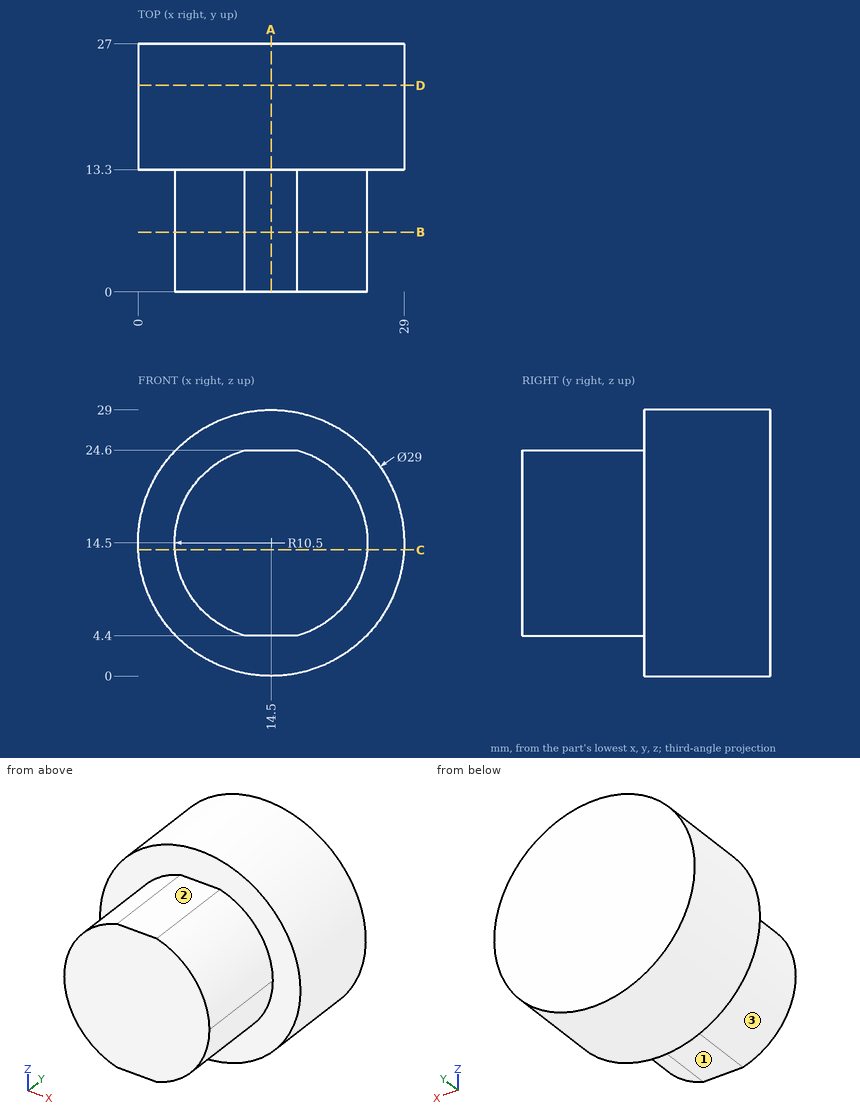
Check sheet for the drawn part. Datum: minimum x, y, z corner. Units: mm. A direction names the side the tool comes from. Coordinates: 2 decimals unless noted, no trailing zeros. Loops run counter-clockwise (first coordinate to the right, second up) from the corner with the lowest first, then second, coordinate; pieces in that order, holes last. Notation, with made-up numbers: (6.5, 74) - (41.5, 74) arc R16 ccw to (41.5, 88) - close; hole circle Ø7 at (82, -4.5). An arc over 180 degrees is marked (long way). Put each result on its own line as item: value.
Item 1: Section check A-A (x = 14.5). Enter the section's corners in (y, z).
Conclusion:
outline: (0, 4.4) - (13.3, 4.4) - (13.3, 0) - (27, 0) - (27, 29) - (13.3, 29) - (13.3, 24.6) - (0, 24.6) - close
Item 2: Section check B-B (y = 6.5). Enter the section's corners in (x, z), then the cut area to 3 significant figures.
Conclusion:
outline: (11.63, 4.4) - (17.37, 4.4) arc R10.5 ccw to (17.37, 24.6) - (11.63, 24.6) arc R10.5 ccw to start
area: 343 mm2
Item 3: Set-up check for the marked faces 1, 2 and 3: record each of +Z, -Z, +X, -X, +Y, -Y from which the full face is reachable in a straight line by a thin tool's end or side.
Conclusion:
face 1: -Z, +X, -X, -Y
face 2: +Z, +X, -X, -Y
face 3: -X, -Y
Item 4: Gauge pin test, flat ends, axial feed: pin 1 Ø4.5 at (x, y) = (14, 5.5) entering from +Z; pin 2 Ø8 at (x, y) = (15, 17) entering from -Z; pin 3 Ø8 at (x, y) = (21, 16.5) entering from +Z; pin 4 Ø2 at (x, y) = (11.5, 3) entering from -Z. Record the tip position at first contact, or that the pin passes through.
Conclusion:
pin 1: stops at z = 24.6
pin 2: stops at z = 0
pin 3: stops at z = 28.78
pin 4: stops at z = 4.4
Item 5: Section check D-D (y = 22.5). Enter the section's corners in (x, z), then the cut area to 3 significant figures.
Conclusion:
outline: circle Ø29 at (14.5, 14.5)
area: 661 mm2
Item 6: Scan lines: line 1 along Y through (x, z) = (2, 14); line 2 along X through (y, z) = (7.75, 11); line 3 along Z through (x, y) = (10.5, 13.25). Record each from-to range of solid material in increasing order.
Conclusion:
line 1: y = 13.3 to 27
line 2: x = 4.6 to 24.4
line 3: z = 4.79 to 24.21
Item 7: Section check C-C (z = 13.75). Enter the section's corners in (x, y).
Conclusion:
outline: (0.02, 13.3) - (4.03, 13.3) - (4.03, 0) - (24.97, 0) - (24.97, 13.3) - (28.98, 13.3) - (28.98, 27) - (0.02, 27) - close
